from build123d import *

# Parameters (mm, degrees)
SKETCH1_W           = 50
SKETCH1_H           = 90
SKETCH1_R           = 3
BOSS_EXTRUDE1_DEPTH = 15
SKETCH2_R           = 3.35
CUT_EXTRUDE1_DEPTH  = 155.757875405
CUT_EXTRUDE2_DEPTH  = 158.718102956
CHAMFER1_SIZE       = 3
FILLET1_R           = 10


with BuildPart() as part:
    # Sketch1 → Boss-Extrude1 (new body)
    with BuildSketch(Plane.XY):
        with Locations((100, 50)):
            Rectangle(SKETCH1_W, SKETCH1_H)
        with Locations((115, 20)):
            Circle(SKETCH1_R, mode=Mode.SUBTRACT)
        with Locations((85, 20)):
            Circle(SKETCH1_R, mode=Mode.SUBTRACT)
        with Locations((115, 80)):
            Circle(SKETCH1_R, mode=Mode.SUBTRACT)
        with Locations((85, 80)):
            Circle(SKETCH1_R, mode=Mode.SUBTRACT)
    extrude(amount=BOSS_EXTRUDE1_DEPTH)

    # Sketch2 → Cut-Extrude1 (cut, through all)
    with BuildSketch(Plane(origin=(0, 95, 0), x_dir=(1, 0, 0), z_dir=(0, 1, 0))):
        with Locations(Location((100, -7.5, 0), (0, 0, 270))):
            Circle(SKETCH2_R)
    extrude(amount=-CUT_EXTRUDE1_DEPTH, mode=Mode.SUBTRACT)

    # Sketch3 → Cut-Extrude2 (cut, through all)
    with BuildSketch(Plane.XY.offset(15)):
        Polygon((90, 70), (90, 74), (110, 74), (110, 70), (110, 30), (90, 30), align=None)
    extrude(amount=-CUT_EXTRUDE2_DEPTH, mode=Mode.SUBTRACT)

    # Chamfer1
    chamfer1_edges = [part.edges().sort_by_distance(p)[0] for p in [
        (75, 50, 15),
        (100, 5, 15),
        (125, 50, 15),
        (100, 95, 15),
    ]]
    chamfer(chamfer1_edges, length=CHAMFER1_SIZE)

    # Fillet1
    fillet1_edges = [part.edges().sort_by_distance(p)[0] for p in [
        (90, 52, 15),
        (110, 52, 15),
    ]]
    fillet(fillet1_edges, radius=FILLET1_R)


solid = part.part
Input: part model. Units: mm. Frame: model coordinates. A direction names the side the tool comes from. Round coordinates to 2 decimals unless told otherwise and drop trailing zeros. Order: outer loops, then holes, each group sorted by start corner. A loop starts at its lowest first (then second) coordinate and runs counter-clockwise, first axis right, second up.
1. Set-up query: faces 4 (the face through (110, 52, 3)), 5 (the face through (100, 23, 15)), 6 (the face through (86.99, 51.69, 12.15)). Return all of +Z, -Z, +X, -X, +Y, -Y with unobstructed straight access to the full face (end or side cutting, diameter ignored); none if empty.
The answers:
face 4: +Z, -Z
face 5: +Z, +X, -X, +Y, -Y
face 6: +Z
2. Cut plane A-A, the plane y = 20. Output: boundary loops of the cut face in (x, z), then the cut area to 3 significant figures.
The answers:
outline: (75, 0) - (82, 0) - (82, 15) - (78, 15) - (75, 12) - close; (88, 0) - (112, 0) - (112, 15) - (88, 15) - close; (118, 0) - (125, 0) - (125, 12) - (122, 15) - (118, 15) - close; hole circle Ø6.7 at (100, 7.5)
area: 526 mm2
3. Cut plane D-D, the plane x = 98. Output: boundary loops of the cut face in (y, z), then the cut area to 3 significant figures.
The answers:
outline: (5, 0) - (30, 0) - (30, 4.81) - (5, 4.81) - close; (5, 10.19) - (30, 10.19) - (30, 15) - (8, 15) - (5, 12) - close; (74, 0) - (95, 0) - (95, 4.81) - (74, 4.81) - close; (74, 10.19) - (95, 10.19) - (95, 12) - (92, 15) - (74, 15) - close
area: 434 mm2
4. Pin query (flat end, axial travel): P1, Ø3.5, axis at x = 115, y = 80, coming from the +Z side. Return the tip coordinate at first contact, or that it passes through.
The answers:
P1: passes through
5. Cut plane B-B, the plane y = 44.5. Output: boundary loops of the cut face in (x, z).
The answers:
outline: (75, 0) - (90, 0) - (90, 5) arc R10 ccw to (80, 15) - (78, 15) - (75, 12) - close; (110, 0) - (125, 0) - (125, 12) - (122, 15) - (120, 15) arc R10 ccw to (110, 5) - close
6. Cut plane C-C, the plane z = 6.25. Output: boundary loops of the cut face in (x, y), then the cut area to 3 significant figures.
The answers:
outline: (75, 5) - (96.89, 5) - (96.89, 30) - (89.92, 30) - (89.92, 74) - (96.89, 74) - (96.89, 95) - (75, 95) - close; (103.11, 5) - (125, 5) - (125, 95) - (103.11, 95) - (103.11, 74) - (110.08, 74) - (110.08, 30) - (103.11, 30) - close; hole circle Ø6 at (85, 20); hole circle Ø6 at (85, 80); hole circle Ø6 at (115, 20); hole circle Ø6 at (115, 80)
area: 3,210 mm2
7. Mould query, pull axis Y, two halves, no side actions, for faces 1 (the face through (100, 93, 14)), 2 (the face through (100, 74, 11)), 3 (the face through (100, 7, 14)). Classes: released by +Y, released by -Y, zero draft, split by the parting line, or undercut.
The answers:
face 1: released by +Y
face 2: undercut
face 3: released by -Y
8. Material intervals for line 1 (Y direction, x = 115, z = 4.5); line 2 (X direction, y = 88.25, z = 7.5); line 3 (Y direction, x = 91.5, z = 7.5), sorted ascending.
The answers:
line 1: y = 5 to 17, 23 to 77, 83 to 95
line 2: x = 75 to 96.65, 103.35 to 125
line 3: y = 5 to 30, 74 to 95
